Read the model definition and answer for the solid it produces. Units are mm, in the model's axes. Round coordinates to 2 decimals unless told otherwise and drop trailing zeros. Loops run counter-clockwise (first coordinate to the right, second up) from the corner with the lowest first, then second, coordinate; pieces in that order, holes last. Notation, with made-up numbers: (55, 59.25) - (101, 59.25) arc R20 cw to (101, 94.25) - close; hole circle Ø1 at (88, 29.5). An arc over 180 degrees is marked (long way). Use CSV: the item, a comma, the result in double quotes. Start each with the question number.
1. Find section B-B (y = 18). Give the vertices of the cut face in (x, z) (1 decimal), and give its area (3 significant figures).
2. Find section A-A (z = 0.4). Give the vertices of the cut face in (x, y).
3. Consider line 1 along X through (y, z) = (13.5, 0.6); line 2 along Z through (x, y) = (0.25, 5); line 3 along Z through (x, y) = (0.3, 4.75). Determine where each line is inside the solid, lowest interval first.
from build123d import *

# Parameters (mm, degrees)
TD_SKETCH_R                   = 0.792499939
TL_FEATURE_DEPTH              = 20.99999991
TDF_STD_SKETCH_W              = 1.604999838
TDF_STD_SKETCH_H              = 1.604999838
TDF_STD_FEATURE_DEPTH         = 22.02988608
ISA_20_STD_FEATURE_DEPTH      = 22.02988608
ISA_20_STD_FEATURE_DEPTH_BACK = 22.02988608
F_10BA_STD_FEATURE_DEPTH      = 22.02988608
F_10BA_STD_FEATURE_DEPTH_BACK = 22.02988608
FRO_STD_FEATURE_DEPTH         = 22.02988608
FRO_STD_FEATURE_DEPTH_BACK    = 22.02988608


with BuildPart() as part:
    # TD_sketch → TL_feature (new body)
    with BuildSketch(Plane(origin=(0, 0, 0), x_dir=(1, 0, 0), z_dir=(0, 1, 0))):
        with Locations(Location((0, 0, 0), (0, 0, 270))):
            Circle(TD_SKETCH_R)
    extrude(amount=TL_FEATURE_DEPTH)

    # TDF_STD_sketch → TDF_STD_feature (cut, through all)
    with BuildSketch(Plane(origin=(0, 0, 0), x_dir=(1, 0, 0), z_dir=(0, 1, 0))):
        with Locations((-1.17799993, 0)):
            Rectangle(TDF_STD_SKETCH_W, TDF_STD_SKETCH_H)
    extrude(amount=TDF_STD_FEATURE_DEPTH, mode=Mode.SUBTRACT)

    # ISA_20_STD_sketch → ISA_20_STD_feature (cut, two sides: drawn at the far end of the back side and taken through both)
    with BuildSketch(Plane(origin=(0, 0, 0), x_dir=(0, 0, -1), z_dir=(1, 0, 0)).offset(-ISA_20_STD_FEATURE_DEPTH_BACK)):
        Polygon((-13.462346915, 73.159859471), (-3.889221277, 20.99999991), (-0.035000057, 0), (0.035000057, 0), (3.889221277, 20.99999991), (13.462346915, 73.159859471), (13.462346915, -32.902305016), (-13.462346915, -32.902305016), align=None)
    extrude(amount=ISA_20_STD_FEATURE_DEPTH + ISA_20_STD_FEATURE_DEPTH_BACK, mode=Mode.SUBTRACT)

    # 10BA_STD_sketch → 10BA_STD_feature (cut, two sides: drawn at the far end of the back side and taken through both)
    with BuildSketch(Plane.XY.offset(-F_10BA_STD_FEATURE_DEPTH_BACK)):
        Polygon((-53.152802148, 0), (-0.375500011, 0), (-0.289499929, 0), (-0.010835963, 0.049135976), (3.683366618, 20.99999991), (12.848048956, 72.975496238), (91.13369141, 2.172017021), (25.132840305, -70.803479216), align=None)
    extrude(amount=F_10BA_STD_FEATURE_DEPTH + F_10BA_STD_FEATURE_DEPTH_BACK, mode=Mode.SUBTRACT)

    # FRO_STD_sketch → FRO_STD_feature (cut, two sides: drawn at the far end of the back side and taken through both)
    with BuildSketch(Plane.XY.offset(-FRO_STD_FEATURE_DEPTH_BACK)):
        with BuildLine():
            Line((-0.375601611, 52.089797523), (-0.375601611, 0.02794))
            ThreePointArc((-0.375601611, 0.02794), (-0.367418174, 0.008183437), (-0.347661611, 0))
            Line((-0.347661611, 0), (51.714195912, 0))
            Line((51.714195912, 0), (-21.91238908, -73.626584992))
            Line((-21.91238908, -73.626584992), (-74.002186603, -21.536787469))
            Line((-74.002186603, -21.536787469), (-0.375601611, 52.089797523))
        make_face()
    extrude(amount=FRO_STD_FEATURE_DEPTH + FRO_STD_FEATURE_DEPTH_BACK, mode=Mode.SUBTRACT)


solid = part.part
Filled sheet:
1,outline,"(-0.4, -0.7) arc R0.8 ccw (long way) to (-0.4, 0.7) - close"
1,area,"1.56 mm²"
2,outline,"(-0.38, 1.99) - (0.33, 1.99) - (0.68, 3.99) - (0.68, 21) - (-0.38, 21) - close"
3,line 1,"x = -0.38 to 0.52"
3,line 2,"z = -0.75 to 0.75"
3,line 3,"z = -0.73 to 0.73"
